Read the model definition and answer for the solid it produces. Units are mm, in the model's axes. A direction names the side the tool comes from. Give positions to 0.01 mm unless a question says otherwise; leave off trailing zeros. Order: outer loops, then holes, each group sorted by start corner. A loop starts at its lowest first (then second) coordinate and runs counter-clockwise, first axis right, second up. Notation, with made-up numbers: (32.25, -39.75) - (91.25, -39.75) arc R27 ccw to (91.25, -20.75) - close; hole circle Ø3 at (39.5, -36.5). An arc over 180 degrees is marked (long way). Write each question's results on one line, items separated by ' | '.
from build123d import *

# Parameters (mm, degrees)
BOSS_EXTRUDE1_DEPTH = 20
RIB1_REACH          = 33.472
SKETCH3_WALL_W      = 79.086555552
SKETCH3_WALL_H      = 3
SKETCH4_R           = 1.65
CUT_EXTRUDE2_DEPTH  = 18
BOSS_EXTRUDE2_START = -2
SKETCH1_4_R         = 1.65
SKETCH1_4_R_2       = 4.5
BOSS_EXTRUDE2_DEPTH = 2


with BuildPart() as part:
    # Sketch1 → Boss-Extrude1 (new body)
    with BuildSketch(Plane(origin=(0, 0, 0), x_dir=(1, 0, 0), z_dir=(0, 1, 0))):
        with BuildLine():
            Line((15.5, 0), (15.5, -10))
            Line((15.5, -10), (25.5, -10))
            Line((25.5, -10), (25.5, -12.5))
            Line((25.5, -12.5), (5, -12.5))
            Line((5, -12.5), (5, -11.456439237))
            ThreePointArc((5, -11.456439237), (0, 12.5), (-5, -11.456439237))
            Line((-5, -11.456439237), (-5, -12.5))
            Line((-5, -12.5), (-25.5, -12.5))
            Line((-25.5, -12.5), (-25.5, -10))
            Line((-25.5, -10), (-15.5, -10))
            Line((-15.5, -10), (-15.5, 0))
            ThreePointArc((-15.5, 0), (0, 15.5), (15.5, 0))
        make_face()
    extrude(amount=BOSS_EXTRUDE1_DEPTH)

    # Sketch3 wall → Rib1 (add, up to next)
    with BuildSketch(Plane(origin=(20.5, 10, 5), x_dir=(0.707106781187, 0, 0.707106781187), z_dir=(0.707106781187, 0, -0.707106781187)), mode=Mode.PRIVATE) as rib1_sk1:
        Rectangle(SKETCH3_WALL_W, SKETCH3_WALL_H)
    rib1_tool1 = extrude(rib1_sk1.sketch, amount=-RIB1_REACH, mode=Mode.PRIVATE) - part.part
    rib1 = rib1_tool1.solids().sort_by_distance((20.5, 10, 5))[0]
    add(rib1)

    # Mirror1: Rib1 across plane
    add(rib1.mirror(Plane(origin=(0, 0, 0), x_dir=(0, 0, 1), z_dir=(1, 0, 0))))

    # Sketch4 → Cut-Extrude2 (cut)
    with BuildSketch(Plane.XY):
        with Locations(Location((20.5, 16, 0), (0, 0, 180))):
            Circle(SKETCH4_R)
        with Locations(Location((20.5, 4, 0), (0, 0, 180))):
            Circle(SKETCH4_R)
    cut_extrude2 = extrude(amount=CUT_EXTRUDE2_DEPTH, mode=Mode.SUBTRACT)

    # Mirror2: Cut-Extrude2 across plane
    add(cut_extrude2.mirror(Plane(origin=(0, 0, 0), x_dir=(0, 0, 1), z_dir=(1, 0, 0))), mode=Mode.SUBTRACT)

    # Sketch1_4 → Boss-Extrude2 (add)
    # profile 1 of 2: a face of its own
    with BuildSketch(Plane(origin=(0, 0, 0), x_dir=(1, 0, 0), z_dir=(0, 1, 0)).offset(BOSS_EXTRUDE2_START)):
        with BuildLine():
            Line((-25.5, -10), (-25.5, -12.5))
            Line((-25.5, -12.5), (-5, -12.5))
            Line((-5, -12.5), (-5, -11.456439237))
            ThreePointArc((-5, -11.456439237), (0, 12.5), (5, -11.456439237))
            Line((5, -11.456439237), (5, -12.5))
            Line((5, -12.5), (25.5, -12.5))
            Line((25.5, -12.5), (25.5, -10))
            Line((25.5, -10), (15.5, -10))
            Line((15.5, -10), (15.5, 0))
            ThreePointArc((15.5, 0), (0, 15.5), (-15.5, 0))
            Line((-15.5, 0), (-15.5, -10))
            Line((-15.5, -10), (-25.5, -10))
        make_face()
    # profile 2 of 2: a face of its own
    with BuildSketch(Plane(origin=(0, 0, 0), x_dir=(1, 0, 0), z_dir=(0, 1, 0)).offset(BOSS_EXTRUDE2_START)):
        with BuildLine():
            Line((-5, -11.456439237), (-5, -12.5))
            Line((-5, -12.5), (5, -12.5))
            Line((5, -12.5), (5, -11.456439237))
            ThreePointArc((5, -11.456439237), (0, 12.5), (-5, -11.456439237))
        make_face()
        with Locations(Location((-8.5, 0, 0), (0, 0, 270))):
            Circle(SKETCH1_4_R, mode=Mode.SUBTRACT)
        with Locations(Location((0, 0, 0), (0, 0, 270))):
            Circle(SKETCH1_4_R_2, mode=Mode.SUBTRACT)
        with Locations(Location((8.5, 0, 0), (0, 0, 270))):
            Circle(SKETCH1_4_R, mode=Mode.SUBTRACT)
    extrude(amount=BOSS_EXTRUDE2_DEPTH)


solid = part.part
(1) Section A-A (x = -20.5) is taken. Give the vertices of the cut face in (y, z).
Conclusion:
outline: (-2, 10) - (2.35, 10) - (2.35, 12.5) - (-2, 12.5) - close; (5.65, 10) - (8.5, 10) - (8.5, 5) - (11.5, 5) - (11.5, 10) - (14.35, 10) - (14.35, 12.5) - (5.65, 12.5) - close; (17.65, 10) - (20, 10) - (20, 12.5) - (17.65, 12.5) - close
(2) Section D-D (y = 9) is taken. Give the vertices of the cut face in (x, z).
Conclusion:
outline: (-25.5, 10) - (-15.5, 0) arc R15.5 ccw to (15.5, 0) - (25.5, 10) - (25.5, 12.5) - (5, 12.5) - (5, 11.46) arc R12.5 cw (long way) to (-5, 11.46) - (-5, 12.5) - (-25.5, 12.5) - close
(3) For faces 1 (the face through (19, 11.5, 7)), 2 (the face through (15.5, 3, 5)), 3 (the face through (-19, 8.5, 7)), determine the directions among +Z, -Z, +X, -X, +Y, -Y from which every point of the face is accessible in a straight line to the end or side of a thin tool.
Conclusion:
face 1: -Z, +X, +Y | face 2: -Z, +X, -Y | face 3: -Z, -X, -Y
(4) Section C-C (z = -3) is taken. Give the vertices of the cut face in (x, y).
Conclusion:
outline: (-15.21, -2) - (-3.35, -2) - (-3.35, 0) - (-12.13, 0) - (-12.13, 20) - (-15.21, 20) - close; (3.35, -2) - (15.21, -2) - (15.21, 20) - (12.13, 20) - (12.13, 0) - (3.35, 0) - close
(5) Consider probe 1 along X at (y, z) = (-1.5, 0); probe 2 along Y at (x, z) = (-20.5, 11.4); probe 3 along X at (y, z) = (3.5, 10.75). Determine where each line is inside the solid, lowest interval first. Write a range as [from, to].
Conclusion:
probe 1: [-15.5, -10.15], [-6.85, -4.5], [4.5, 6.85], [10.15, 15.5] | probe 2: [-2, 2.35], [5.65, 14.35], [17.65, 20] | probe 3: [-25.5, -22.07], [-18.93, -6.38], [6.38, 18.93], [22.07, 25.5]
(6) Section B-B (y = 4) is taken. Give the vertices of the cut face in (x, z).
Conclusion:
outline: (-25.5, 10) - (-22.15, 10) - (-22.15, 12.5) - (-25.5, 12.5) - close; (-18.85, 10) - (-15.5, 10) - (-15.5, 0) arc R15.5 ccw to (15.5, 0) - (15.5, 10) - (18.85, 10) - (18.85, 12.5) - (5, 12.5) - (5, 11.46) arc R12.5 cw (long way) to (-5, 11.46) - (-5, 12.5) - (-18.85, 12.5) - close; (22.15, 10) - (25.5, 10) - (25.5, 12.5) - (22.15, 12.5) - close
(7) Each of these flat-tipped pins is pushed along its axis until it touches: pin 1 (6 mm diameter, centred on y = 1, z = -1, fed in from +X); pin 2 (6 mm diameter, centred on x = 6, z = -2, fed in from +Y); pin 3 (3 mm diameter, centred on y = 11.5, z = -5.5, fed in from -X) (3 decimals); pin 4 (2 mm diameter, centred on x = -20.5, y = 16, fed in from -Z). Where does it stop, or does it pass through?
Conclusion:
pin 1: x = 15.5 | pin 2: y = 0 | pin 3: x = -14.975 | pin 4: through
(8) The mould has two halves that part along X. Classify faces 4 (the face through (1.352, -1.014, 4.292)), 5 (the face through (0.48, 9.86, -12.49)), 6 (the face through (15.5, 16, 5)), 7 (the face through (19, 8.5, 7)): pulls with the +X half, pulls with the -X half, needs draft (parallel to the pull), parting line crosses it, or undercut.
Conclusion:
face 4: undercut | face 5: undercut | face 6: pulls with the +X half | face 7: needs draft
